The drawing under review shows one solid part. Ordinate dimensions are in mm from its lowest x, y, z. A direction names the side the tool comes from. Give positions to 0.01 mm unless a question says otherwise; leave off trailing zeros. Order: outer loops, then holes, each group sorted by start corner. A loop starts at its lowest first (then second) coordinate and runs counter-clockwise, first axis right, second up. Notation, with made-up numbers: (78, 33) -> (119, 33) arc R16 cw to (119, 60) -> close; hole circle Ø10 at (61.5, 66). An arc over 180 degrees is marked (long way). One line per item, written item: value. Start each with the question number.
1) Consider section A-A (y = 12.5). State the section outline as (x, z) points.
2) Consider section C-C (z = 7). State the section outline as (x, y) points (1 decimal).
3) Consider section B-B (x = 1.35). State the section outline as (y, z) points, plus the area to 3 significant figures.
4) Consider section D-D (y = 6.75). State the section outline as (x, z) points.
5) Tool access review of the marked faces 1, 2 and 3: name each direction out of +Z, -Z, +X, -X, +Y, -Y from which nothing blocks a thin tool from reaching the whole face with its end or side.
6) Wall thickness on line 1 along Z through (x, y) = (1.4, 8); line 2 along Y through (x, z) = (2, 0.4); line 3 along Y through (x, z) = (1.3, 1) (1 decimal): over which ranges is each line inside the solid? List them lowest first. Write a range as from..to.
7) For pin 1 (2 mm diameter, centred on x = 5, y = 3, fed in from +Z); pin 2 (1 mm diameter, centred on x = 5, z = 7.5, fed in from -Y) (1 decimal); pin 3 (1 mm diameter, centred on x = 4.5, z = 7, fed in from +Y), all flat-tipped, find the tip position at first contact; note any pin that passes through.
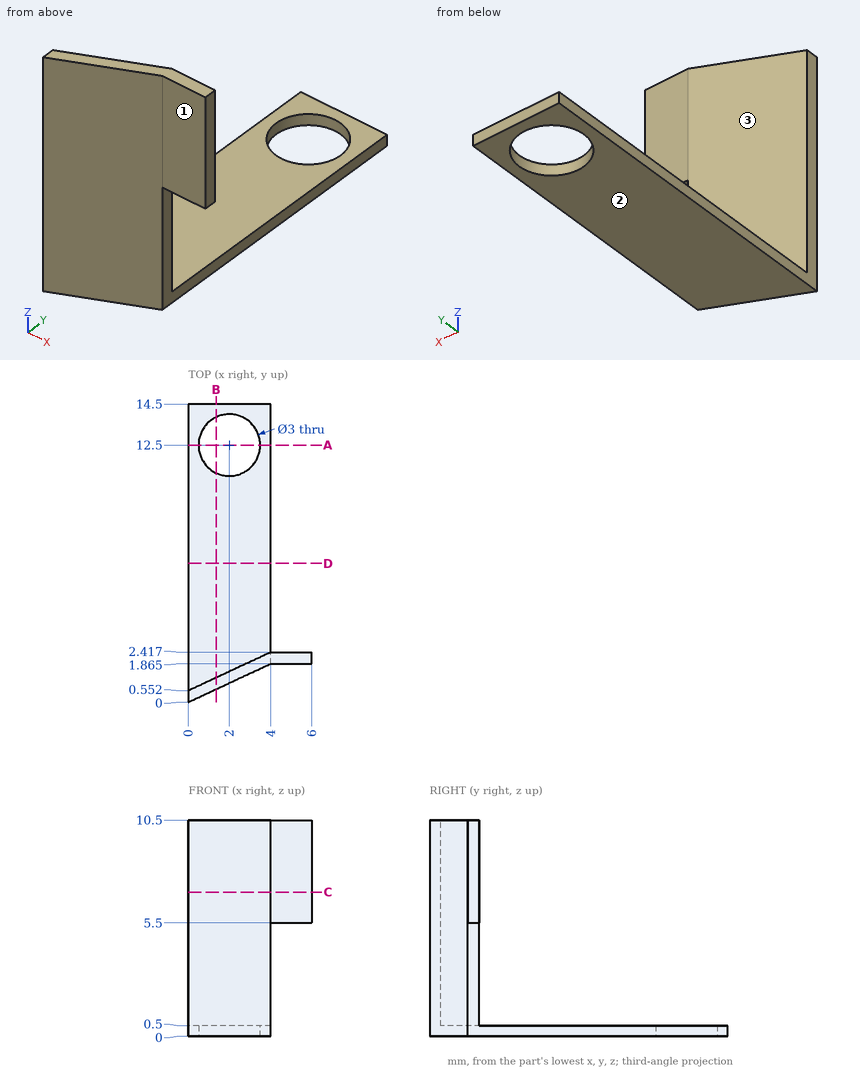
Checked values:
1. outline: (0, 0) -> (0.5, 0) -> (0.5, 0.5) -> (0, 0.5) -> close; (3.5, 0) -> (4, 0) -> (4, 0.5) -> (3.5, 0.5) -> close
2. outline: (0, 0) -> (4, 1.9) -> (6, 1.9) -> (6, 2.4) -> (4, 2.4) -> (0, 0.6) -> close
3. outline: (0.63, 0) -> (11.15, 0) -> (11.15, 0.5) -> (1.18, 0.5) -> (1.18, 10.5) -> (0.63, 10.5) -> close; (13.85, 0) -> (14.5, 0) -> (14.5, 0.5) -> (13.85, 0.5) -> close
3. area: 11.1 mm^2
4. outline: (0, 0) -> (4, 0) -> (4, 0.5) -> (0, 0.5) -> close
5. face 1: +Z, -Z, +X, -Y
5. face 2: -Z, +X, -X, +Y, -Y
5. face 3: +Z, -X, +Y
6. line 1: z = 0..0.5
6. line 2: y = 0.93..11, 14..14.5
6. line 3: y = 0.6..1.2
7. pin 1: stops at z = 10.5
7. pin 2: stops at y = 1.9
7. pin 3: stops at y = 2.42
